Design review of the part built by this model. Coordinates are the model's own, in mm. A direction names the side the tool comes from. Round coordinates to 2 decimals unless told otherwise and drop trailing zeros. Loops run counter-clockwise (first coordinate to the right, second up) from the corner with the lowest first, then second, coordinate; pieces in that order, holes last. Notation, with made-up numbers: (77, 11.25) - (115, 11.25) arc R20 ccw to (115, 21.25) - close; hole circle Ø5 at (81.25, 82). An arc over 180 degrees is marked (long way). Return JSON: item names as keys, results as strings. Group by question number.
(1) Wall thickness on L1, parallel to Y at x = 0, z = 85; L2, parallel to X at y = 0, z = 60; L3, parallel to Z at x = -14.5, y = -14.5: over which ranges is each line inside the solid? List them lowest first. Write a range as [from, to].
(2) We need section B-B, the plane y = 17.5. Give the number of separate pieces and of enclosed holes in the cut face, and give its area (3 significant figures).
(3) We need section A-A, the plane z = 25. Write out the cut boundary in (x, y), and give its area (3 significant figures).
(4) Clearance check with flat-ended pins moving along their axes: pin 1 (2 mm diameter, centred on x = 7, z = 37, fed in from +Y); pin 2 (2.5 mm diameter, centred on x = 0, y = -17.5, fed in from -Z); pin 3 (5 mm diameter, centred on y = 1.5, z = 76.5, fed in from +X). State where each tip first meets the part, or that it passes through.
(5) The part is to be moulded in two halves that separate along Y. For faces 1 (the cylindrical face through (10.382, -19.961, 88.523)), 2 (the cylindrical face through (0.208, 15.914, 87.814)), 3 (the flat face through (-4, -14, 6.45)), say which applies: pulls with the +Y half, pulls with the -Y half, needs draft (parallel to the pull), parting line crosses it, or undercut.
(6) For faces 4 (the flat face through (3, -11, 0)), 5 (the cylindrical face through (-15.4, 0.07, 7.46)), 6 (the flat face through (-4, -14, 8.45)), 7 (the cylindrical face through (0.208, 19.086, 7.464)), 8 (the cylindrical face through (15.9, 0.07, 87.81)), list the 3-axis set-ups (+Z, -Z, +X, -X, +Y, -Y) from which the entire face can be reached by the end or side of a thin tool; tool diameter is ignored.
from build123d import *

# Parameters (mm, degrees)
SKETCH2_R               = 11
SKETCH2_R_2             = 9.45
BOSS_EXTRUDE2_DEPTH     = 88.1
BOSS_EXTRUDE3_START     = -5
SKETCH3_R               = 22.5
SKETCH3_R_2             = 11
BOSS_EXTRUDE3_DEPTH     = 5
FILLET1_R               = 10
CUT_EXTRUDE1_START      = -3
SKETCH4_R               = 11
SKETCH4_R_2             = 9.45
CUT_EXTRUDE1_DEPTH      = 3
SKETCH7_R               = 14.31
SKETCH7_R_2             = 11
BOSS_EXTRUDE6_DEPTH     = 20
SKETCH8_R               = 11
CUT_EXTRUDE3_DEPTH      = 7
SKETCH10_R              = 21.1
SKETCH10_R_2            = 14.31
BOSS_EXTRUDE8_DEPTH     = 2
CUT_EXTRUDE4_DEPTH      = 88.631173106
CUT_EXTRUDE4_DEPTH_BACK = 2
SKETCH11_R              = 1.6
CHAMFER5_SIZE           = 5
CUT_EXTRUDE5_START      = -10
SKETCH12_R              = 1.6
CUT_EXTRUDE5_DEPTH      = 10
SKETCH13_R              = 22.5
SKETCH13_R_2            = 13
SKETCH13_R_3            = 1.6
BOSS_EXTRUDE9_DEPTH     = 6


with BuildPart() as part:
    # Sketch2 → Boss-Extrude2 (new body)
    with BuildSketch(Plane.XY):
        Circle(SKETCH2_R)
        Circle(SKETCH2_R_2, mode=Mode.SUBTRACT)
    extrude(amount=BOSS_EXTRUDE2_DEPTH)

    # Sketch3 → Boss-Extrude3 (add)
    with BuildSketch(Plane.XY.offset(88.1).offset(BOSS_EXTRUDE3_START)):
        Circle(SKETCH3_R)
        Circle(SKETCH3_R_2, mode=Mode.SUBTRACT)
    extrude(amount=BOSS_EXTRUDE3_DEPTH)

    # Fillet1
    fillet1_edges = [part.edges().sort_by_distance(p)[0] for p in [
        (-11, 0, 83.1),
    ]]
    fillet(fillet1_edges, radius=FILLET1_R)

    # Sketch4 → Cut-Extrude1 (cut)
    with BuildSketch(Plane.XY.offset(88.1).offset(CUT_EXTRUDE1_START)):
        Circle(SKETCH4_R)
        Circle(SKETCH4_R_2, mode=Mode.SUBTRACT)
    extrude(amount=CUT_EXTRUDE1_DEPTH, mode=Mode.SUBTRACT)

    # Sketch7 → Boss-Extrude6 (add)
    with BuildSketch(Plane(origin=(0, 0, 0), x_dir=(-1, 0, 0), z_dir=(0, 0, -1))):
        Circle(SKETCH7_R)
        Circle(SKETCH7_R_2, mode=Mode.SUBTRACT)
    extrude(amount=-BOSS_EXTRUDE6_DEPTH)

    # Sketch8 → Cut-Extrude3 (cut)
    with BuildSketch(Plane(origin=(0, 0, 0), x_dir=(-1, 0, 0), z_dir=(0, 0, -1))):
        Circle(SKETCH8_R)
    extrude(amount=-CUT_EXTRUDE3_DEPTH, mode=Mode.SUBTRACT)

    # Sketch10 → Boss-Extrude8 (add)
    with BuildSketch(Plane(origin=(0, 0, 6.45), x_dir=(-1, 0, 0), z_dir=(0, 0, -1))):
        Circle(SKETCH10_R)
        Circle(SKETCH10_R_2, mode=Mode.SUBTRACT)
    extrude(amount=-BOSS_EXTRUDE8_DEPTH)

    # Sketch11 → Cut-Extrude4 (cut, two sides: drawn at the far end of the back side and taken through both)
    with BuildSketch(Plane(origin=(0, 0, 6.45), x_dir=(-1, 0, 0), z_dir=(0, 0, -1)).offset(-CUT_EXTRUDE4_DEPTH_BACK)):
        with Locations((0, 17.5)):
            Circle(SKETCH11_R)
        with Locations((17, 0)):
            Circle(SKETCH11_R)
        with Locations((-0.5, -17)):
            Circle(SKETCH11_R)
        with Locations((-17.5, 0.5)):
            Circle(SKETCH11_R)
    extrude(amount=CUT_EXTRUDE4_DEPTH + CUT_EXTRUDE4_DEPTH_BACK, mode=Mode.SUBTRACT)

    # Chamfer5
    # the kernel refuses this chamfer: 5 mm, written as the material it takes off along each edge
    with BuildSketch(Plane(origin=(0, 0, 20), x_dir=(-1, 0, 0), z_dir=(0, -1, 0))) as chamfer5_piece_1_section:
        Polygon((14.31 - CHAMFER5_SIZE, 0), (14.31, CHAMFER5_SIZE), (14.31, 0), align=None)
    chamfer5_piece_1 = revolve(axis=Axis((0, 0, 20), (0, 0, -1)), mode=Mode.PRIVATE)
    chamfer5_piece_1 = chamfer5_piece_1 - Plane(origin=(0, 0, 16.654544166), x_dir=(1, 0, 0), z_dir=(0, 0, -1)) * Cylinder(11, 58, mode=Mode.PRIVATE)
    add(chamfer5_piece_1, mode=Mode.SUBTRACT)

    # Sketch12 → Cut-Extrude5 (cut)
    with BuildSketch(Plane.XY.offset(88.1).offset(CUT_EXTRUDE5_START)):
        with Locations(Location((0, 17.5, 0), (0, 0, 180))):
            Circle(SKETCH12_R)
        with Locations((17.5, 0)):
            Circle(SKETCH12_R)
        with Locations((0, -17.5)):
            Circle(SKETCH12_R)
        with Locations((-17.5, 0)):
            Circle(SKETCH12_R)
    extrude(amount=CUT_EXTRUDE5_DEPTH, mode=Mode.SUBTRACT)

    # Sketch13 → Boss-Extrude9 (add)
    with BuildSketch(Plane.XY.offset(88.1)):
        Circle(SKETCH13_R)
        Circle(SKETCH13_R_2, mode=Mode.SUBTRACT)
        with Locations((-17.5, 0)):
            Circle(SKETCH13_R_3, mode=Mode.SUBTRACT)
        with Locations((17.5, 0)):
            Circle(SKETCH13_R_3, mode=Mode.SUBTRACT)
        with Locations((0, -17.5)):
            Circle(SKETCH13_R_3, mode=Mode.SUBTRACT)
        with Locations(Location((0, 17.5, 0), (0, 0, 180))):
            Circle(SKETCH13_R_3, mode=Mode.SUBTRACT)
    extrude(amount=BOSS_EXTRUDE9_DEPTH)


solid = part.part
Solutions:
{
 "1": {"L1": "[-22.5, -19.1], [-15.9, -9.45], [9.45, 15.9], [19.1, 22.5]", "L2": "[-11, -9.45], [9.45, 11]", "L3": "[6.45, 8.45], [83.09, 94.1]"},
 "2": {"separate pieces": "4", "enclosed holes": "0", "area": "322 mm^2"},
 "3": {"outline": "circle Ø22 at (0, 0); hole circle Ø18.9 at (0, 0)", "area": "99.6 mm^2"},
 "4": {"pin 1": "y = 9.22", "pin 2": "z = 6.45", "pin 3": "x = 12.86"},
 "5": {"face 1": "parting line crosses it", "face 2": "undercut", "face 3": "needs draft"},
 "6": {"face 4": "-Z, +X, -X, +Y, -Y", "face 5": "-Z", "face 6": "none", "face 7": "+Z, -Z", "face 8": "+Z"}
}
